Drawing for the job (mm, zero at the part's lowest x, y, z). A direction names the side the tool comes from. Give positions to 0.01 mm unless a question says otherwise; leave off trailing zeros. Write each loop counter-clockwise with the first axis right and the second up, starting at its lowest first coordinate (ties: lowest second). Pieces come first, ordered by that corner, then holes. Notation, with made-up numbers: (34, -7) - (71, -7) arc R33 cw to (71, 30) - close; hole circle Ø5 at (-2, 52). An arc over 180 degrees is marked (long way). Use CSV: the item, a comma, the result in double quotes.
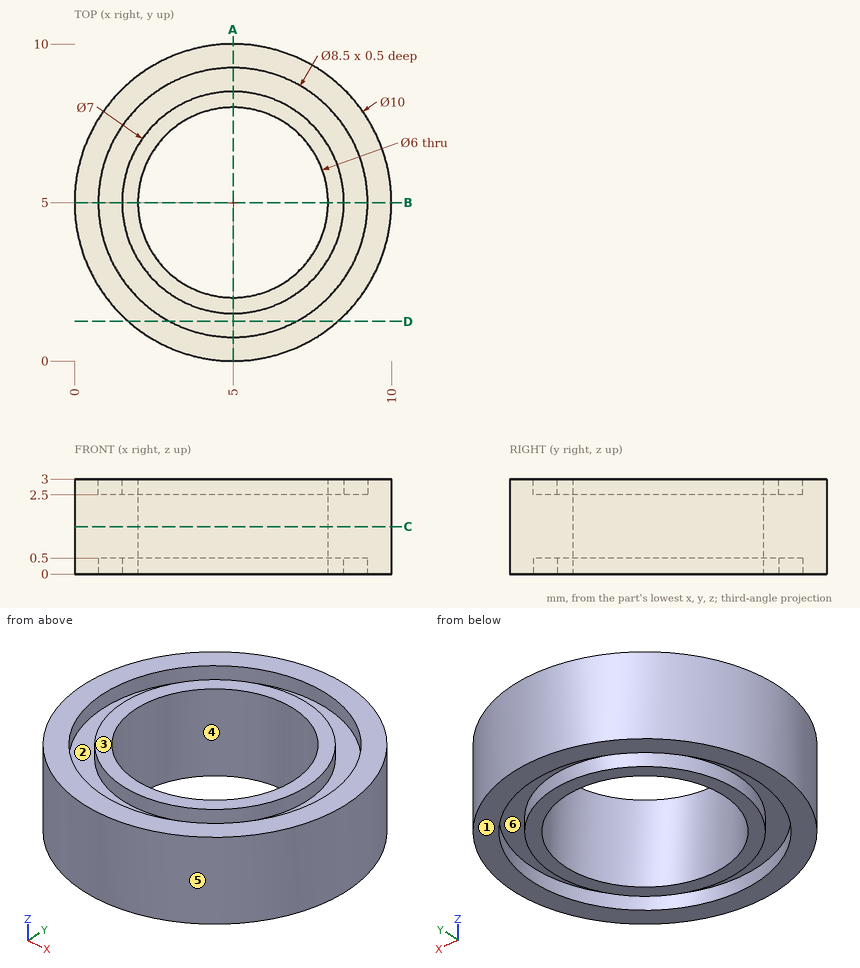
(1) Saw through at D-D, the plane y = 1.25. List the corners of the cut face in (x, z), then the cut area to 3 significant figures.
Checked values:
outline,"(1.69, 0) - (3, 0) - (3, 0.5) - (7, 0.5) - (7, 0) - (8.31, 0) - (8.31, 3) - (7, 3) - (7, 2.5) - (3, 2.5) - (3, 3) - (1.69, 3) - close"
area,"15.8 mm^2"
(2) Pull direction Y, two halves, no side cores. Call the marked faces 3, 4, 5 and 6: released by +Y, released by -Y, zero draft, split by the parting line, or undercut.
Checked values:
face 3,"zero draft"
face 4,"undercut"
face 5,"split by the parting line"
face 6,"undercut"
(3) Flat gauge pins, fed straight in: P1, Ø5.5, axis at x = 5, y = 5, coming from the -Z side; P2, Ø1.5, axis at x = 2.5, z = 2, coming from the +Y side. Where does each tip first touch, or does it go through?
Checked values:
P1,"passes through"
P2,"stops at y = 9.68"
(4) Saw through at A-A, the plane x = 5. List the corners of the cut face in (y, z).
Checked values:
outline,"(0, 0) - (0.75, 0) - (0.75, 0.5) - (1.5, 0.5) - (1.5, 0) - (2, 0) - (2, 3) - (1.5, 3) - (1.5, 2.5) - (0.75, 2.5) - (0.75, 3) - (0, 3) - close; (8, 0) - (8.5, 0) - (8.5, 0.5) - (9.25, 0.5) - (9.25, 0) - (10, 0) - (10, 3) - (9.25, 3) - (9.25, 2.5) - (8.5, 2.5) - (8.5, 3) - (8, 3) - close"
(5) 3-axis set-ups, long thin cutter, end or side, ignore diameter. For the marked faces 1 and 2: which of +Z, -Z, +X, -X, +Y, -Y reach the whole face in a straight line?
Checked values:
face 1,"-Z, +X, -X, +Y, -Y"
face 2,"+Z"
(6) Saw through at C-C, the plane z = 1.5. List the corners of the cut face in (x, y).
Checked values:
outline,"circle Ø10 at (5, 5); hole circle Ø6 at (5, 5)"
(7) Wall check: probe 1 along Y at (x, z) = (5, 2.8); probe 2 along Y at (x, z) = (5, 0.9); probe 3 along Z at (x, y) = (1.5, 7.25). Give the ranges that are in metal, low to high. Write a range as [from, to].
Checked values:
probe 1,"y = [0, 0.75], [1.5, 2], [8, 8.5], [9.25, 10]"
probe 2,"y = [0, 2], [8, 10]"
probe 3,"z = [0.5, 2.5]"
